from build123d import *

# Parameters (mm, degrees)
F1_DEPTH = 25
F2_R     = 100
F4_DEPTH = 25
F6_DEPTH = 25
F8_DEPTH = 539
F9_R     = 15


with BuildPart() as f1:
    # F0 (on Top) → F1 (new body)
    with BuildSketch(Plane.XY):
        Polygon((0, 0), (0, 600), (-500, 600), (-500, 0), (0, -500), (800, -500), (800, 0), align=None)
    extrude(amount=F1_DEPTH)

    # F2
    f2_edges = [f1.edges().sort_by_distance(p)[0] for p in [
        (-500, 0, 12.5),
        (0, -500, 12.5),
    ]]
    fillet(f2_edges, radius=F2_R)

    # F3 (on face) → F4 (join)
    with BuildSketch(Plane.XY.offset(25)):
        with BuildLine():
            Line((-525, 625), (-525, 41.4213562373))
            ThreePointArc((-525, 41.4213562373), (-515.4849415639, -6.4140728083), (-488.3883476483, -46.966991411))
            Line((-488.3883476483, -46.966991411), (-46.966991411, -488.3883476483))
            ThreePointArc((-46.966991411, -488.3883476483), (-6.4140728083, -515.4849415639), (41.4213562373, -525))
            Line((41.4213562373, -525), (825, -525))
            Line((825, -525), (825, 25))
            Line((825, 25), (25, 25))
            Line((25, 25), (25, 625))
            Line((25, 625), (-525, 625))
        make_face()
    extrude(amount=F4_DEPTH)

    # F5 (on face) → F6 (join)
    with BuildSketch(Plane.XY.offset(50)):
        with BuildLine():
            Line((-550, 650), (-550, 41.4213562373))
            ThreePointArc((-550, 41.4213562373), (-538.5819298767, -15.9811586175), (-506.066017178, -64.6446609407))
            Line((-506.066017178, -64.6446609407), (-64.6446609407, -506.066017178))
            ThreePointArc((-64.6446609407, -506.066017178), (-15.9811586175, -538.5819298767), (41.4213562373, -550))
            Line((41.4213562373, -550), (850, -550))
            Line((850, -550), (850, 50))
            Line((850, 50), (50, 50))
            Line((50, 50), (50, 650))
            Line((50, 650), (-550, 650))
        make_face()
    extrude(amount=F6_DEPTH)

    # F7 (on face) → F8 (cut)
    with BuildSketch(Plane(origin=(0, 0, 0), x_dir=(1, 0, 0), z_dir=(0, 0, -1))):
        Polygon((800, 759.8769068718), (800, 0), (0, 0), (0, -600), (-650.8337855339, -600), (-650.8337855339, -840.3587818146), (869.2708611488, -840.3587818146), (869.2708611488, 0), (869.2708611488, 759.8769068718), align=None)
    extrude(amount=-F8_DEPTH, mode=Mode.SUBTRACT)

    # F9
    f9_edges = [f1.edges().sort_by_distance(p)[0] for p in [
        (420.710678, -500, 0),
        (420.710678, -525, 25),
        (420.710678, -550, 50),
        (3.153013, -492.387953, 0),
        (-6.414073, -515.484942, 25),
        (-15.981159, -538.58193, 50),
        (-250, -250, 0),
        (-267.67767, -267.67767, 25),
        (-285.355339, -285.355339, 50),
        (-492.387953, 3.153013, 0),
        (-515.484942, -6.414073, 25),
        (-538.58193, -15.981159, 50),
        (-500, 320.710678, 0),
        (-525, 320.710678, 25),
        (-550, 320.710678, 50),
    ]]
    fillet(f9_edges, radius=F9_R)


solid = f1.part
The listing builds one solid part. Answer for the finished solid, in the listing's coordinates (mm). A direction names the side the tool comes from. Coordinates: 2 decimals unless noted, no trailing zeros. Write each loop counter-clockwise with the first axis right and the second up, starting at its lowest first coordinate (ties: lowest second). Pieces come first, ordered by that corner, then holes. Notation, with made-up numbers: M 87,28 L 91,28 A24 ccw 91,53 Z; hole C -31.5,55 d5. An arc over 180 degrees is marked long. Use one line per item in the form item = value.
Item 1: For faces 1 (the face through (-253, -247, 20)), 2 (the face through (6, -55, 0)), 3 (the face through (0, 296, 37)), determine the directions among +Z, -Z, +X, -X, +Y, -Y from which every point of the face is accessible in a straight line to the end or side of a thin tool.
Model answer:
face_1 = -Z, -X, -Y
face_2 = -Z, +X, -X, +Y, -Y
face_3 = +Z, -Z, +X, +Y
Item 2: Find section A-A, the plane y = 207. Give the vertices of the cut face in (x, z), plus the area to 3 significant figures.
Model answer:
outline = M -550,65 A15 ccw -535,50 L -525,50 L -525,40 A15 ccw -510,25 L -500,25 L -500,15 A15 ccw -485,0 L 0,0 L 0,75 L -550,75 Z
area = 39,200 mm2
Item 3: Find the intervals of material crossed by probe 1 along X at (y, z) = (-25, 44); probe 2 along X at (y, z) = (548, 71.5); probe 3 along Y at (x, z) = (302, 19.5), in increasing order.
Model answer:
probe_1 = -505.89 to 800
probe_2 = -550 to 0
probe_3 = -500 to 0
Item 4: Given P1, Ø8, axis at x = -214.5, z = 10, coming from the -Y side; P2, Ø4, axis at x = -317, z = 52, coming from the -Y side; P3, Ø22.5, axis at y = 175.5, z = 34, coming from the +X side, each flat-ended and moving along its own axis, determine where each tip first touches the part or whether it passes through.
Model answer:
P1 = -288.63
P2 = -247.5
P3 = 0
